Source: CAD feature listing. Evaluate the final solid. Frame: model axes, mm. A direction names the side the tool comes from. Round coordinates to 2 decimals unless told otherwise and drop trailing zeros. Loops run counter-clockwise (first coordinate to the right, second up) from the corner with the lowest first, then second, coordinate; pieces in that order, holes last. Notation, with made-up numbers: (47, -19.5) -> (56, -19.5) arc R35 cw to (56, 14.5) -> close; hole circle Ø5 at (11, -15). An arc over 180 degrees is marked (long way). Put each result on its own line as item: value. Start each with the question number.
1. Cut plane C-C (y = -5.75). Return the cut outline in (x, z).
2. Set-up query: faces 1 (the flat face through (0, -4, 3.2)), 2 (the flat face through (0, -5, 0.25)), 3 (the flat face through (-4.25, -3.6, 1.5)). Return all of +Z, -Z, +X, -X, +Y, -Y with unobstructed straight access to the full face (end or side cutting, diameter ignored); none if empty.
3. Draft query along Z for faces 4 (the cylindrical face through (4.3, -4.4, 0.4)), 5 (the flat face through (4.25, -3.6, 1.5)), 6 (the cylindrical face through (-4.199, -3.599, 2.915)), 7 (the flat face through (4.5, -4, 2)). Return one class per face: pulls with the +Z half, pulls with the -Z half, needs draft (parallel to the pull), parting line crosses it, or undercut.
4. Material intervals for L1, parallel to X at y = -3.25, z = 1.4; L2, parallel to Z at x = -3.25, y = -6, sorted ascending.
5. Cut plane D-D (y = -1.5). Return the cut outline in (x, z), then the cut area to 3 significant figures.
6. Cut plane A-A (z = 1.35). Return the cut outline in (x, y).
7. Cut plane B-B (x = -1.5). Return the cut outline in (y, z), then the cut area to 3 significant figures.
```python
from build123d import *

# Parameters (mm, degrees)
BOX067_W               = 8.5
BOX067_H               = 2.95
BOX067_DEPTH           = 3
FILLET011_R            = 0.75
EXTRUDE016_DEPTH       = 7.3
CUT016_PLACEMENT_ANGLE = 90


with BuildPart() as clone037:
    # Box067 → Box067 (new body)
    with BuildSketch(Plane(origin=(-4.25, 0, 0), x_dir=(1, 0, 0), z_dir=(0, 0, 1))):
        with Locations((4.25, 1.475)):
            Rectangle(BOX067_W, BOX067_H)
    extrude(amount=BOX067_DEPTH)

    # Fillet011
    fillet011_edges = [clone037.edges().sort_by_distance(p)[0] for p in [
        (-4.25, 2.95, 1.5),
        (4.25, 2.95, 1.5),
    ]]
    fillet(fillet011_edges, radius=FILLET011_R)


with BuildPart() as shield:
    # Sketch017 → Extrude016 (new body)
    with BuildSketch(Plane.XY):
        with BuildLine():
            Line((-3.5, 3.2), (3.5, 3.2))
            ThreePointArc((4.5, 2.2), (4.207107, 2.907107), (3.5, 3.2))
            Line((4.5, 2.2), (4.5, 1))
            ThreePointArc((3.5, 0), (4.207107, 0.292893), (4.5, 1))
            Line((-3.5, 0), (3.5, 0))
            ThreePointArc((-4.5, 1), (-4.207107, 0.292893), (-3.5, 0))
            Line((-4.5, 2.2), (-4.5, 1))
            ThreePointArc((-3.5, 3.2), (-4.207107, 2.907107), (-4.5, 2.2))
        make_face()
        with BuildLine():
            Line((-3.5, 2.95), (3.5, 2.95))
            ThreePointArc((4.25, 2.2), (4.03033, 2.73033), (3.5, 2.95))
            Line((4.25, 2.2), (4.25, 1))
            ThreePointArc((3.5, 0.25), (4.03033, 0.46967), (4.25, 1))
            Line((3.5, 0.25), (-3.5, 0.25))
            ThreePointArc((-4.25, 1), (-4.03033, 0.46967), (-3.5, 0.25))
            Line((-4.25, 1), (-4.25, 2.2))
            ThreePointArc((-3.5, 2.95), (-4.03033, 2.73033), (-4.25, 2.2))
        make_face(mode=Mode.SUBTRACT)
    extrude(amount=EXTRUDE016_DEPTH)

    # Cut016: cut Clone037
    add(clone037.part, mode=Mode.SUBTRACT)


with BuildPart() as shield_1:
    # Cut016 placement: moved
    add(shield.part.rotate(Axis((0, 0, 0), (1, 0, 0)), CUT016_PLACEMENT_ANGLE))


solid = shield_1.part
```
Solution:
1. outline: (-4.5, 1) arc R1 ccw to (-3.5, 0) -> (3.5, 0) arc R1 ccw to (4.5, 1) -> (4.5, 2.2) arc R1 ccw to (3.5, 3.2) -> (-3.5, 3.2) arc R1 ccw to (-4.5, 2.2) -> close; hole (-4.25, 1) arc R0.75 ccw to (-3.5, 0.25) -> (3.5, 0.25) arc R0.75 ccw to (4.25, 1) -> (4.25, 2.2) arc R0.75 ccw to (3.5, 2.95) -> (-3.5, 2.95) arc R0.75 ccw to (-4.25, 2.2) -> close
2. face 1: +Z, +X, -X, +Y, -Y
2. face 2: +Y, -Y
2. face 3: +Y
3. face 4: pulls with the -Z half
3. face 5: undercut
3. face 6: pulls with the +Z half
3. face 7: needs draft
4. L1: x = -4.5 to -4.25, 4.25 to 4.5
4. L2: z = 0 to 0.25, 2.95 to 3.2
5. outline: (-4.5, 1) arc R1 ccw to (-4.25, 0.34) -> (-4.25, 2.2) arc R0.75 cw to (-3.5, 2.95) -> (3.5, 2.95) arc R0.75 cw to (4.25, 2.2) -> (4.25, 0.34) arc R1 ccw to (4.5, 1) -> (4.5, 2.2) arc R1 ccw to (3.5, 3.2) -> (-3.5, 3.2) arc R1 ccw to (-4.5, 2.2) -> close
5. area: 3.26 mm^2
6. outline: (-4.5, -7.3) -> (-4.25, -7.3) -> (-4.25, 0) -> (-4.5, 0) -> close; (4.25, -7.3) -> (4.5, -7.3) -> (4.5, 0) -> (4.25, 0) -> close
7. outline: (-7.3, 0) -> (-3, 0) -> (-3, 0.25) -> (-7.3, 0.25) -> close; (-7.3, 2.95) -> (0, 2.95) -> (0, 3.2) -> (-7.3, 3.2) -> close
7. area: 2.90 mm^2
